Source: three-view drawing plus pictorial views. Frame: mm from the lowest corner of the part. A direction names the side the tool comes from. Coordinates: 2 decimals unless noted, no trailing zeros. Loops run counter-clockwise (first coordinate to the right, second up) from the corner with the lowest first, then second, coordinate; pieces in that order, holes last. Notation, with made-up numbers: M 52,52.5 L 56,52.5 A8 ccw 56,66.5 Z; hole C 31,-32 d8. An arc over 180 degrees is marked long. Use a Markdown table: item, result. Add a question column.
1. Line query: L1, parallel to Y at x = 118, z = 31; L2, parallel to X at y = 39.5, z = 16; L3, parallel to Z at x = 74, y = 51.5. Output: solid intervals per line, ascending. Write a range as [from, to].
2. Section C-C on x = 98. Output: boundary loops of the cut face in (y, z).
3. Draft query along Y for the marked faces 1, 2 and 3. Return one class per face: +Y half, -Y half, draft (parallel to the pull), parting line (faces both ways), or undercut.
4. Set-up query: the marked faces 4 and 5. Return all of +Z, -Z, +X, -X, +Y, -Y with unobstructed straight access to the full face (end or side cutting, diameter ignored); none if empty.
5. Section A-A on y = 45. Output: boundary loops of the cut face in (x, z), then the cut area to 3 significant figures.
6. Section B-B on z = 18. Output: boundary loops of the cut face in (x, y).
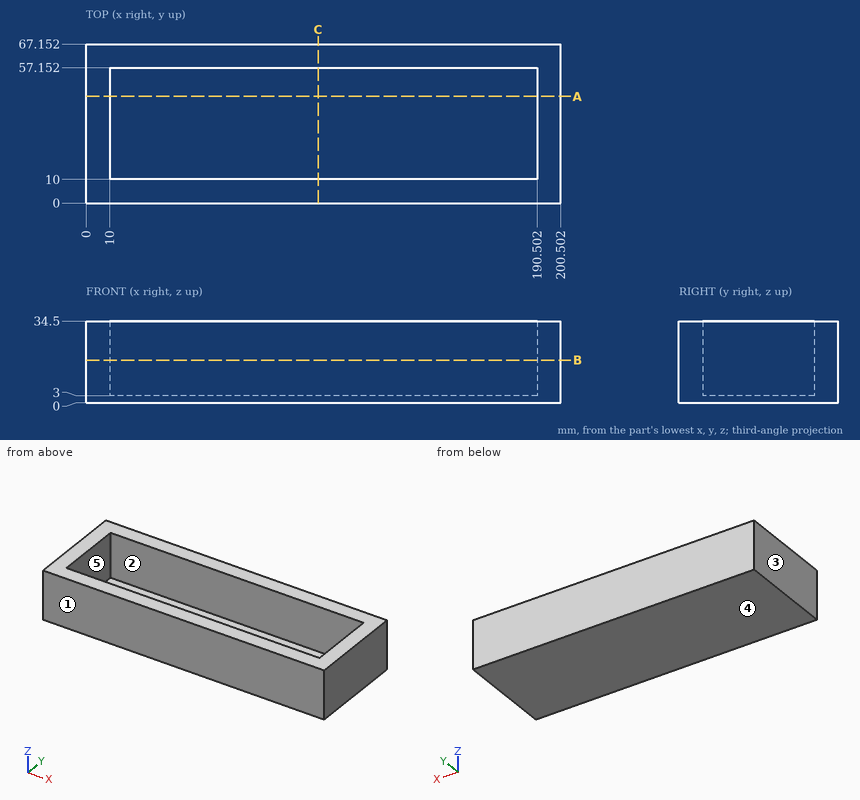
Answers below:
| question | item | result |
|---|---|---|
| 1 | L1 | y = [0, 10], [57.15, 67.15] |
| 1 | L2 | x = [0, 10], [190.5, 200.5] |
| 1 | L3 | z = [0, 3] |
| 2 | outline | M 0,0 L 67.15,0 L 67.15,34.5 L 57.15,34.5 L 57.15,3 L 10,3 L 10,34.5 L 0,34.5 Z |
| 3 | face 1 | -Y half |
| 3 | face 2 | undercut |
| 3 | face 3 | draft |
| 4 | face 4 | -Z, +X, -X, +Y, -Y |
| 4 | face 5 | +Z |
| 5 | outline | M 0,0 L 200.5,0 L 200.5,34.5 L 190.5,34.5 L 190.5,3 L 10,3 L 10,34.5 L 0,34.5 Z |
| 5 | area | 1,230 mm² |
| 6 | outline | M 0,0 L 200.5,0 L 200.5,67.15 L 0,67.15 Z; hole M 10,10 L 190.5,10 L 190.5,57.15 L 10,57.15 Z |
